Geometry check sheet. Reference: the model listing, model coordinates, mm. A direction names the side the tool comes from. Give positions to 0.01 mm unless a question says otherwise; leave off trailing zeros. Loops run counter-clockwise (first coordinate to the right, second up) from the corner with the lowest first, then second, coordinate; pieces in that order, holes last. Notation, with made-up numbers: (-35, -32.75) -> (10, -32.75) arc R15 cw to (10, -20.75) -> close; hole circle Ø10 at (15.25, 75). An arc over 180 degrees is marked (long way). One line per item, written item: value. Start each with the question number.
(1) Draft check along X on faces 1 (the face through (46, -22, -67)), 2 (the face through (43.025, -11.534, -67.042)), 3 (the face through (71.503, -8, -67)). Enter one of: pulls with the +X half, pulls with the -X half, needs draft (parallel to the pull), parting line crosses it, or undercut.
(2) Scan lines: line 1 along X through (y, z) = (6, -67.7); line 2 along Y through (x, z) = (63.5, -67.7); line 3 along X through (y, z) = (-10.8, -67.75). Record each from-to range of solid material in increasing order. Write a range as from..to.
(3) Sectioned sample at A-A, the plane y = -4. Record the cut outline in (x, z), then the cut area to 3 significant figures.
(4) Sectioned sample at B-B, the plane x = 63. Record the cut outline in (y, z), then the cut area to 3 significant figures.
(5) Sectioned sample at D-D, the plane y = 7. Record the cut outline in (x, z).
(6) Sectioned sample at C-C, the plane z = -69.1. Record the cut outline in (x, y) (3 decimals).
(7) Gauge pin test, flat ends, axial feed: pin 1 Ø1.8 at (y, z) = (-18, -67) entering from +X; pin 2 Ø3 at (x, z) = (66, -68.5) entering from +Y; pin 3 Ø1.8 at (y, z) = (-18, -68) entering from -X. Record the tip position at first contact, or that the pin passes through.
(8) Tool access check on faces 4 (the face through (43.065, 5, -67)), 5 (the face through (63.941, -19, -67)), 6 (the face through (49.615, 5, -67)), 7 (the face through (63.941, 5, -67)), 8 (the face through (43.065, -19, -67)). Record the directions out of +Z, -Z, +X, -X, +Y, -Y that give a thin tool (end or side, any length) a straight path to the whole face; none if there is none.
from build123d import *

# Parameters (mm, degrees)
SZKIC1_W                      = 36
SZKIC1_H                      = 16
DODANIE_WYCI_GNI_CIE1_DEPTH   = 6
WYTNIJ_WYCI_GNI_CIE1_DEPTH    = 6
SZKIC3_R                      = 1.55
WYTNIJ_WYCI_GNI_CIE2_DEPTH    = 74.51650454
SZKIC5_W                      = 6.55
SZKIC5_H                      = 6
DODANIE_WYCI_GNI_CIE2_DEPTH   = 6
DODANIE_WYCI_GNI_CIE2_2_DEPTH = 6
SZKIC7_W                      = 6.55
SZKIC7_H                      = 6
DODANIE_WYCI_GNI_CIE3_DEPTH   = 10


with BuildPart() as part:
    # Szkic1 → Dodanie-wyciągnięcie1 (new body)
    with BuildSketch(Plane.XY.offset(-64.000000001)):
        with Locations((53.502982034, -8)):
            Rectangle(SZKIC1_W, SZKIC1_H)
    extrude(amount=-DODANIE_WYCI_GNI_CIE1_DEPTH)

    # Szkic2 → Wytnij-wyciągnięcie1 (cut)
    with BuildSketch(Plane.XY.offset(-70.000000001)):
        with BuildLine():
            Line((49.614537615, -16), (49.614537615, -14.730541148))
            Line((49.614537615, -14.730541148), (49.186780246, -15.145805693))
            ThreePointArc((49.186780246, -15.145805693), (49.13517548, -15.093936528), (49.084193998, -15.041454619))
            ThreePointArc((49.084193998, -15.041454619), (53.502982034, -4.675), (57.921770071, -15.041454619))
            ThreePointArc((57.921770071, -15.041454619), (57.867648174, -15.097128633), (57.812824874, -15.152112096))
            Line((57.812824874, -15.152112096), (57.391426454, -14.730541148))
            Line((57.391426454, -14.730541148), (57.391426454, -16))
            Line((57.391426454, -16), (49.614537615, -16))
        make_face()
    extrude(amount=WYTNIJ_WYCI_GNI_CIE1_DEPTH, mode=Mode.SUBTRACT)

    # Szkic3 → Wytnij-wyciągnięcie2 (cut, through all)
    with BuildSketch(Plane(origin=(0, 0, -70.000000001), x_dir=(-1, 0, 0), z_dir=(0, 0, -1))):
        with Locations((-62.502982034, -4)):
            Circle(SZKIC3_R)
        with Locations((-44.502982034, -4)):
            Circle(SZKIC3_R)
        with Locations((-44.502982034, -12)):
            Circle(SZKIC3_R)
        with Locations((-62.502982034, -12)):
            Circle(SZKIC3_R)
    extrude(amount=-WYTNIJ_WYCI_GNI_CIE2_DEPTH, mode=Mode.SUBTRACT)


with BuildPart() as body_2:
    # Szkic5 → Dodanie-wyciągnięcie2 (new body)
    with BuildSketch(Plane.XZ.offset(16)):
        with Locations((60.666426454, -67.000000001)):
            Rectangle(SZKIC5_W, SZKIC5_H)
    extrude(amount=DODANIE_WYCI_GNI_CIE2_DEPTH)


with BuildPart() as body_3:
    # Szkic5 → Dodanie-wyci_gni_cie2 2 (new body)
    with BuildSketch(Plane.XZ.offset(16)):
        with Locations((46.339537615, -67.000000001)):
            Rectangle(SZKIC5_W, SZKIC5_H)
    extrude(amount=DODANIE_WYCI_GNI_CIE2_2_DEPTH)


with BuildPart() as part_1:
    add(part.part)

    # Połącz6: union body 2
    add(body_2.part)

    # Szkic7 → Dodanie-wyciągnięcie3 (add)
    with BuildSketch(Plane(origin=(0, 0, 0), x_dir=(1, 0, 0), z_dir=(0, 1, 0))):
        with Locations((60.666426454, 67.000000001)):
            Rectangle(SZKIC7_W, SZKIC7_H)
        with Locations((46.339537615, 67.000000001)):
            Rectangle(SZKIC7_W, SZKIC7_H)
    extrude(amount=DODANIE_WYCI_GNI_CIE3_DEPTH)


with BuildPart() as body_3_1:
    add(body_3.part)

    # Połącz8: union part
    add(part_1.part)


solid = body_3_1.part
Calculated:
1. face 1: needs draft
1. face 2: undercut
1. face 3: pulls with the +X half
2. line 1: x = 43.06..49.61, 57.39..63.94
2. line 2: y = -22..-13.19, -10.81..-5.19, -2.81..10
2. line 3: x = 35.5..43.52, 45.48..47.38, 59.63..61.52, 63.48..71.5
3. outline: (35.5, -70) -> (42.95, -70) -> (42.95, -64) -> (35.5, -64) -> close; (46.05, -70) -> (60.95, -70) -> (60.95, -64) -> (46.05, -64) -> close; (64.05, -70) -> (71.5, -70) -> (71.5, -64) -> (64.05, -64) -> close
3. area: 179 mm2
4. outline: (-22, -70) -> (-13.47, -70) -> (-13.47, -64) -> (-22, -64) -> close; (-10.53, -70) -> (-5.47, -70) -> (-5.47, -64) -> (-10.53, -64) -> close; (-2.53, -70) -> (10, -70) -> (10, -64) -> (-2.53, -64) -> close
4. area: 157 mm2
5. outline: (43.06, -70) -> (49.61, -70) -> (49.61, -64) -> (43.06, -64) -> close; (57.39, -70) -> (63.94, -70) -> (63.94, -64) -> (57.39, -64) -> close
6. outline: (35.503, -16) -> (43.065, -16) -> (43.065, -22) -> (49.615, -22) -> (49.615, -14.731) -> (49.187, -15.146) arc R6.125 cw to (49.084, -15.041) arc R6.125 cw (long way) to (57.813, -15.152) -> (57.391, -14.731) -> (57.391, -22) -> (63.941, -22) -> (63.941, -16) -> (71.503, -16) -> (71.503, 0) -> (63.941, 0) -> (63.941, 10) -> (57.391, 10) -> (57.391, 0) -> (49.615, 0) -> (49.615, 10) -> (43.065, 10) -> (43.065, 0) -> (35.503, 0) -> close; hole circle Ø3.1 at (44.503, -12); hole circle Ø3.1 at (44.503, -4); hole circle Ø3.1 at (62.503, -12); hole circle Ø3.1 at (62.503, -4)
7. pin 1: stops at x = 63.94
7. pin 2: stops at y = 0
7. pin 3: stops at x = 43.06
8. face 4: +Z, -Z, -X, +Y
8. face 5: +Z, -Z, +X, -Y
8. face 6: +Z, -Z, +Y
8. face 7: +Z, -Z, +X, +Y
8. face 8: +Z, -Z, -X, -Y
